```python
from build123d import *

# Parameters (mm, degrees)
CROQUIS1_W              = 300
CROQUIS1_H              = 270
SALIENTE_EXTRUIR1_DEPTH = 5
CROQUIS2_W              = 5
CROQUIS2_H              = 259.826620651
CROQUIS2_W_2            = 260.893012834
CROQUIS2_H_2            = 6.115910783
SALIENTE_EXTRUIR2_DEPTH = 20
CROQUIS3_R              = 3.417677686
CROQUIS3_R_2            = 4.551592261
CORTAR_EXTRUIR1_DEPTH   = 330.015197217
CROQUIS4_R              = 3
SALIENTE_EXTRUIR3_DEPTH = 20
CROQUIS5_R              = 3.841776338
CROQUIS5_R_2            = 4.628228364
CORTAR_EXTRUIR2_DEPTH   = 20


with BuildPart() as part:
    # Croquis1 → Saliente-Extruir1 (new body)
    with BuildSketch(Plane.XY):
        Rectangle(CROQUIS1_W, CROQUIS1_H)
    extrude(amount=SALIENTE_EXTRUIR1_DEPTH)

    # Croquis2 → Saliente-Extruir2 (add)
    with BuildSketch(Plane.XY.offset(5)):
        with Locations((-146.5, -0.015689121)):
            Rectangle(CROQUIS2_W, CROQUIS2_H)
        with Locations((146.5, -0.015689121)):
            Rectangle(CROQUIS2_W, CROQUIS2_H)
        with Locations((0.463771802, 131.942044608)):
            Rectangle(CROQUIS2_W_2, CROQUIS2_H_2)
    extrude(amount=SALIENTE_EXTRUIR2_DEPTH)

    # Croquis3 → Cortar-Extruir1 (cut, through all)
    with BuildSketch(Plane.ZY.offset(149)):
        with Locations(Location((15.036244293, 116.297685092, 0), (0, 0, 90))):
            Circle(CROQUIS3_R)
        with Locations(Location((15.036244293, -98.258041649, 0), (0, 0, 90))):
            Circle(CROQUIS3_R_2)
    extrude(amount=-CORTAR_EXTRUIR1_DEPTH, mode=Mode.SUBTRACT)

    # Croquis4 → Saliente-Extruir3 (add)
    with BuildSketch(Plane.XY.offset(5)):
        with Locations((-10, 0)):
            Circle(CROQUIS4_R)
        with Locations((10, 0)):
            Circle(CROQUIS4_R)
    extrude(amount=SALIENTE_EXTRUIR3_DEPTH)

    # Croquis5 → Cortar-Extruir2 (cut)
    with BuildSketch(Plane(origin=(0, 135, 0), x_dir=(1, 0, 0), z_dir=(0, 1, 0))):
        with Locations(Location((-76.809917119, -13.943258858, 0), (0, 0, 180))):
            Circle(CROQUIS5_R)
        with Locations(Location((84.376229975, -13.943258858, 0), (0, 0, 180))):
            Circle(CROQUIS5_R_2)
    extrude(amount=-CORTAR_EXTRUIR2_DEPTH, mode=Mode.SUBTRACT)


solid = part.part
```
Part model, mm, in its own coordinate system. A direction names the side the tool comes from. Give positions to 0.01 mm unless a question says otherwise; leave off trailing zeros. Loops run counter-clockwise (first coordinate to the right, second up) from the corner with the lowest first, then second, coordinate; pieces in that order, holes last. Notation, with made-up numbers: M 77,51.5 L 122,51.5 A17 cw 122,67.5 Z; hole C -8,-14.5 d9. An arc over 180 degrees is marked long. Return JSON: item names as keys, results as strings.
1) Pull direction Y, two halves, no side cores. Call faces 5 (the face through (-80.474, 131.985, 15.097)), 6 (the face through (-2, 135, 12)), 7 (the face through (146.465, -94.054, 16.78)): released by +Y, released by -Y, zero draft, split by the parting line, or undercut.
Calculated:
{"face 5": "zero draft", "face 6": "released by +Y", "face 7": "undercut"}
2) 3-axis set-ups, long thin cutter, end or side, ignore diameter. For faces 1 (the face through (-149, -2, 15)), 2 (the face through (149, -2, 15)), 3 (the face through (-129.983, 132, 15)), 4 (the face through (146.465, 119.558, 14.01)): which of +Z, -Z, +X, -X, +Y, -Y reach the whole face in a straight line?
Calculated:
{"face 1": "+Z, -X, +Y, -Y", "face 2": "+Z, +X, +Y, -Y", "face 3": "+Z, +Y, -Y", "face 4": "+X, -X"}
3) Drill centre lines: line 1 (X direction, y = 88.5, z = 8.5); line 2 (Y direction, x = 127.5, z = 14.5); line 3 (Z direction, x = 108, y = 113). Where is each one in solid material? Low to high.
Calculated:
{"line 1": "x = -149 to -144, 144 to 149", "line 2": "y = 128.88 to 135", "line 3": "z = 0 to 5"}
4) Saw through at A-A, the plane y = 37. List the corners of the cut face in (x, z), then the cut area to 3 significant figures.
Calculated:
{"outline": "M -150,0 L 150,0 L 150,5 L 149,5 L 149,25 L 144,25 L 144,5 L -144,5 L -144,25 L -149,25 L -149,5 L -150,5 Z", "area": "1,700 mm2"}
5) Flat gauge pins, fed straight in: pin 1 Ø9 at (y, z) = (116.3, 15.04) entering from -X; pin 2 Ø9 at (x, z) = (-76.81, 13.94) entering from -Y; pin 3 Ø3 at (y, z) = (130.5, 19.5) entering from +X. Where does each tip first touch, or does it go through?
Calculated:
{"pin 1": "stops at x = -149", "pin 2": "stops at y = 128.88", "pin 3": "stops at x = 149"}
6) Saw through at B-B, the plane x = -23. List the corners of the cut face in (y, z), then the cut area to 3 significant figures.
Calculated:
{"outline": "M -135,0 L 135,0 L 135,25 L 128.88,25 L 128.88,5 L -135,5 Z", "area": "1,470 mm2"}
